Verification items for this drawing (mm, ordinates from the low corner). Round coordinates to 2 decimals unless told otherwise and drop trailing zeros. Order: outer loops, then holes, each group sorted by start corner. A loop starts at its lowest first (then second) coordinate and runs counter-clockwise, first axis right, second up. Notation, with made-up numbers: (-11.5, -35.75) -> (40.5, -35.75) arc R21 ccw to (40.5, -16.75) -> close; hole circle Ø8 at (63, 65.5). An arc over 180 degrees is marked (long way). Return JSON: item names as keys, results as strings. Group by question number.
Item 1: Sectioned sample at C-C on y = 2.25. Record the cut outline in (x, z) (3 decimals), plus the area to 3 significant figures.
Item 2: Draft check along Z on the marked faces 1, 2 and 3. Enter one of: pulls with the +Z half, pulls with the -Z half, needs draft (parallel to the pull), parting line crosses it, or undercut.
Item 3: Depth check by flat-ended pin: pin 1 Ø5 at (x, z) = (18.5, 16) entering from -Y. Enter the tip coordinate at first touch or a pass-through.
Item 4: Sectioned sample at B-B on x = 37. Record the cut outline in (y, z) (3 decimals), plus the area to 3 significant figures.
Item 5: Sectioned sample at A-A on z = 2.5. Record the cut outline in (x, y), plus the area to 3 significant figures.
Item 6: Scan lines: probe 1 along Z at (x, y) = (6.6, 4.25); probe 2 along Z at (x, y) = (37, 5.75) (3 decimals); probe 3 along X at (y, z) = (11.5, 2). Record each from-to range of solid material in increasing order. Write a range as from..to.
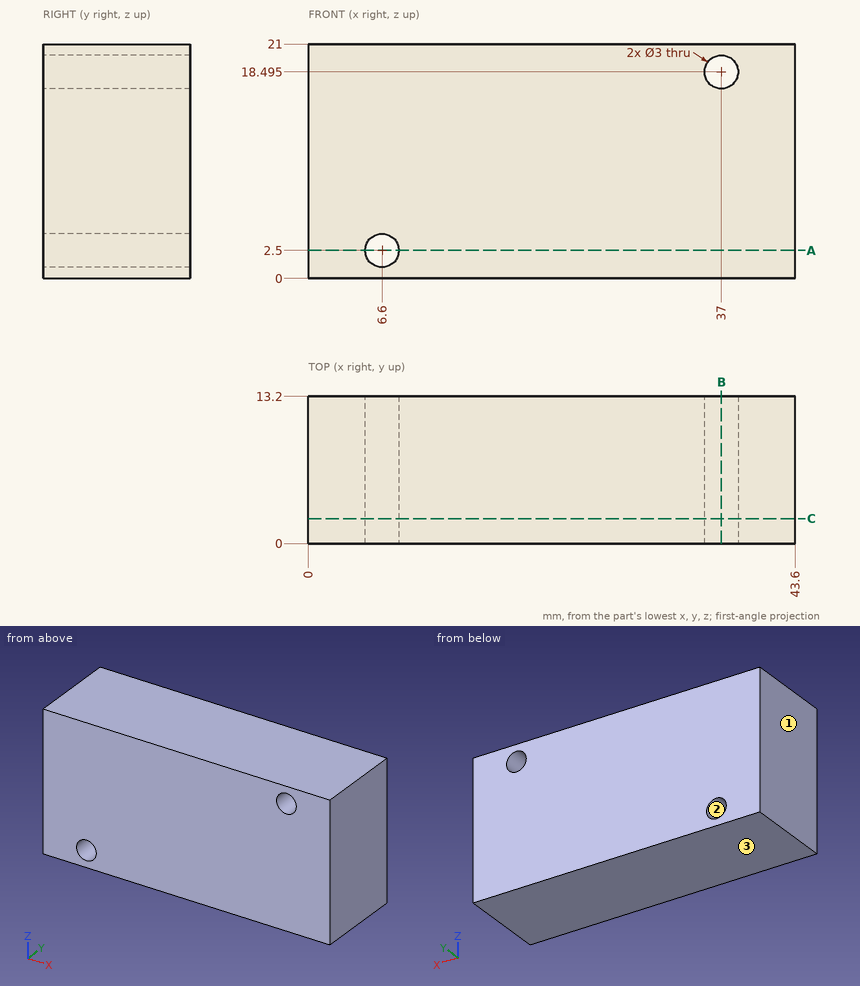
Recorded:
{
 "1": {"outline": "(0, 0) -> (43.6, 0) -> (43.6, 21) -> (0, 21) -> close; hole circle Ø3 at (6.6, 2.5); hole circle Ø3 at (37, 18.495)", "area": "901 mm²"},
 "2": {"face 1": "needs draft", "face 2": "undercut", "face 3": "pulls with the -Z half"},
 "3": {"pin 1": "y = 0"},
 "4": {"outline": "(0, 0) -> (13.2, 0) -> (13.2, 16.995) -> (0, 16.995) -> close; (0, 19.995) -> (13.2, 19.995) -> (13.2, 21) -> (0, 21) -> close", "area": "238 mm²"},
 "5": {"outline": "(0, 0) -> (5.1, 0) -> (5.1, 13.2) -> (0, 13.2) -> close; (8.1, 0) -> (43.6, 0) -> (43.6, 13.2) -> (8.1, 13.2) -> close", "area": "536 mm²"},
 "6": {"probe 1": "0..1, 4..21", "probe 2": "0..16.995, 19.995..21", "probe 3": "0..5.19, 8.01..43.6"}
}
